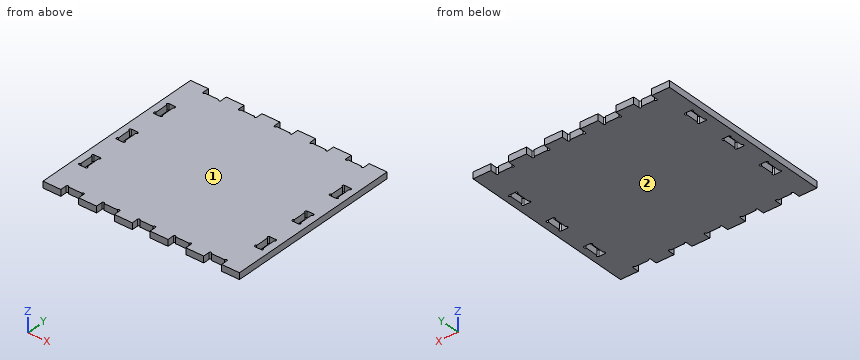
from build123d import *

# Parameters (mm, degrees)
ESTRUSIONE_ESTRUSIONE1_DEPTH = 18
TAGLIO_ESTRUSIONE1_DEPTH     = 115
TAGLIO_ESTRUSIONE2_DEPTH     = 258
TAGLIO_ESTRUSIONE3_DEPTH     = 723
TAGLIO_ESTRUSIONE4_DEPTH     = 160
TAGLIO_ESTRUSIONE5_DEPTH     = 190
TAGLIO_ESTRUSIONE6_DEPTH     = 231


with BuildPart() as part:
    # Schizzo2 → Estrusione-Estrusione1 (new body)
    with BuildSketch(Plane.XY):
        with BuildLine():
            Line((-275, -250), (-275, 250))
            Line((-275, 250), (-225, 250))
            Line((-225, 250), (-225, 232))
            ThreePointArc((-225, 232), (-221.825, 228.825), (-218.65, 232))
            Line((-218.65, 232), (-181.35, 232))
            ThreePointArc((-181.35, 232), (-178.175, 228.825), (-175, 232))
            Line((-175, 232), (-175, 250))
            Line((-175, 250), (-125, 250))
            Line((-125, 250), (-125, 232))
            ThreePointArc((-125, 232), (-121.825, 228.825), (-118.65, 232))
            Line((-118.65, 232), (-81.35, 232))
            ThreePointArc((-81.35, 232), (-78.175, 228.825), (-75, 232))
            Line((-75, 232), (-75, 250))
            Line((-75, 250), (-25, 250))
            Line((-25, 250), (-25, 232))
            ThreePointArc((-25, 232), (-21.825, 228.825), (-18.65, 232))
            Line((-18.65, 232), (18.65, 232))
            ThreePointArc((18.65, 232), (21.825, 228.825), (25, 232))
            Line((25, 232), (25, 250))
            Line((25, 250), (75, 250))
            Line((75, 250), (75, 232))
            ThreePointArc((75, 232), (78.175, 228.825), (81.35, 232))
            Line((81.35, 232), (118.65, 232))
            ThreePointArc((118.65, 232), (121.825, 228.825), (125, 232))
            Line((125, 232), (125, 250))
            Line((125, 250), (175, 250))
            Line((175, 250), (175, 232))
            ThreePointArc((175, 232), (178.175, 228.825), (181.35, 232))
            Line((181.35, 232), (218.65, 232))
            ThreePointArc((218.65, 232), (221.825, 228.825), (225, 232))
            Line((225, 232), (225, 250))
            Line((225, 250), (275, 250))
            Line((275, 250), (275, -250))
            Line((275, -250), (225, -250))
            Line((225, -250), (225, -232))
            ThreePointArc((225, -232), (221.825, -228.825), (218.65, -232))
            Line((218.65, -232), (181.35, -232))
            ThreePointArc((181.35, -232), (178.175, -228.825), (175, -232))
            Line((175, -232), (175, -250))
            Line((175, -250), (125, -250))
            Line((125, -250), (125, -232))
            ThreePointArc((125, -232), (121.825, -228.825), (118.65, -232))
            Line((118.65, -232), (81.35, -232))
            ThreePointArc((81.35, -232), (78.175, -228.825), (75, -232))
            Line((75, -232), (75, -250))
            Line((75, -250), (25, -250))
            Line((25, -250), (25, -232))
            ThreePointArc((25, -232), (21.825, -228.825), (18.65, -232))
            Line((18.65, -232), (-18.65, -232))
            ThreePointArc((-18.65, -232), (-21.825, -228.825), (-25, -232))
            Line((-25, -232), (-25, -250))
            Line((-25, -250), (-75, -250))
            Line((-75, -250), (-75, -232))
            ThreePointArc((-75, -232), (-78.175, -228.825), (-81.35, -232))
            Line((-81.35, -232), (-118.65, -232))
            ThreePointArc((-118.65, -232), (-121.825, -228.825), (-125, -232))
            Line((-125, -232), (-125, -250))
            Line((-125, -250), (-175, -250))
            Line((-175, -250), (-175, -232))
            ThreePointArc((-175, -232), (-178.175, -228.825), (-181.35, -232))
            Line((-181.35, -232), (-218.65, -232))
            ThreePointArc((-218.65, -232), (-221.825, -228.825), (-225, -232))
            Line((-225, -232), (-225, -250))
            Line((-225, -250), (-275, -250))
        make_face()
    extrude(amount=ESTRUSIONE_ESTRUSIONE1_DEPTH)

    # Schizzo2<4> → Taglio-Estrusione1 (cut)
    with BuildSketch(Plane.XY):
        with BuildLine():
            Line((237, 145.65), (237, 108.35))
            ThreePointArc((237, 108.35), (233.825, 105.175), (237, 102))
            Line((237, 102), (255, 102))
            ThreePointArc((255, 102), (258.175, 105.175), (255, 108.35))
            Line((255, 108.35), (255, 145.65))
            ThreePointArc((255, 145.65), (258.175, 148.825), (255, 152))
            Line((255, 152), (237, 152))
            ThreePointArc((237, 152), (233.825, 148.825), (237, 145.65))
        make_face()
    extrude(amount=TAGLIO_ESTRUSIONE1_DEPTH, mode=Mode.SUBTRACT)

    # Schizzo2<5> → Taglio-Estrusione2 (cut)
    with BuildSketch(Plane.XY):
        with BuildLine():
            Line((255, -18.65), (255, 18.65))
            ThreePointArc((255, 18.65), (258.175, 21.825), (255, 25))
            Line((255, 25), (237, 25))
            ThreePointArc((237, 25), (233.825, 21.825), (237, 18.65))
            Line((237, 18.65), (237, -18.65))
            ThreePointArc((237, -18.65), (233.825, -21.825), (237, -25))
            Line((237, -25), (255, -25))
            ThreePointArc((255, -25), (258.175, -21.825), (255, -18.65))
        make_face()
    extrude(amount=TAGLIO_ESTRUSIONE2_DEPTH, mode=Mode.SUBTRACT)

    # Schizzo2<7> → Taglio-Estrusione3 (cut)
    with BuildSketch(Plane.XY):
        with BuildLine():
            Line((255, -152), (237, -152))
            ThreePointArc((237, -152), (233.825, -148.825), (237, -145.65))
            Line((237, -145.65), (237, -108.35))
            ThreePointArc((237, -108.35), (233.825, -105.175), (237, -102))
            Line((237, -102), (255, -102))
            ThreePointArc((255, -102), (258.175, -105.175), (255, -108.35))
            Line((255, -108.35), (255, -145.65))
            ThreePointArc((255, -145.65), (258.175, -148.825), (255, -152))
        make_face()
    extrude(amount=TAGLIO_ESTRUSIONE3_DEPTH, mode=Mode.SUBTRACT)

    # Schizzo2<8> → Taglio-Estrusione4 (cut)
    with BuildSketch(Plane.XY):
        with BuildLine():
            Line((-255, 152), (-237, 152))
            ThreePointArc((-237, 152), (-233.825, 148.825), (-237, 145.65))
            Line((-237, 145.65), (-237, 108.35))
            ThreePointArc((-237, 108.35), (-233.825, 105.175), (-237, 102))
            Line((-237, 102), (-255, 102))
            ThreePointArc((-255, 102), (-258.175, 105.175), (-255, 108.35))
            Line((-255, 108.35), (-255, 145.65))
            ThreePointArc((-255, 145.65), (-258.175, 148.825), (-255, 152))
        make_face()
    extrude(amount=TAGLIO_ESTRUSIONE4_DEPTH, mode=Mode.SUBTRACT)

    # Schizzo2<9> → Taglio-Estrusione5 (cut)
    with BuildSketch(Plane.XY):
        with BuildLine():
            Line((-255, 25), (-237, 25))
            ThreePointArc((-237, 25), (-233.825, 21.825), (-237, 18.65))
            Line((-237, 18.65), (-237, -18.65))
            ThreePointArc((-237, -18.65), (-233.825, -21.825), (-237, -25))
            Line((-237, -25), (-255, -25))
            ThreePointArc((-255, -25), (-258.175, -21.825), (-255, -18.65))
            Line((-255, -18.65), (-255, 18.65))
            ThreePointArc((-255, 18.65), (-258.175, 21.825), (-255, 25))
        make_face()
    extrude(amount=TAGLIO_ESTRUSIONE5_DEPTH, mode=Mode.SUBTRACT)

    # Schizzo2<10> → Taglio-Estrusione6 (cut)
    with BuildSketch(Plane.XY):
        with BuildLine():
            Line((-237, -145.65), (-237, -108.35))
            ThreePointArc((-237, -108.35), (-233.825, -105.175), (-237, -102))
            Line((-237, -102), (-255, -102))
            ThreePointArc((-255, -102), (-258.175, -105.175), (-255, -108.35))
            Line((-255, -108.35), (-255, -145.65))
            ThreePointArc((-255, -145.65), (-258.175, -148.825), (-255, -152))
            Line((-255, -152), (-237, -152))
            ThreePointArc((-237, -152), (-233.825, -148.825), (-237, -145.65))
        make_face()
    extrude(amount=TAGLIO_ESTRUSIONE6_DEPTH, mode=Mode.SUBTRACT)


solid = part.part
Work out the finished part from the listing and answer in its coordinate system (mm). Face numbers are marked on the shaded views. Give positions to 0.01 mm unless a question says otherwise; leave off trailing zeros. Loops run counter-clockwise (first coordinate to the right, second up) from the corner with the lowest first, then second, coordinate; pieces in that order, holes last. Notation, with made-up numbers: (29, -21) - (86, -21) arc R21 ccw to (86, 17) - close; hole circle Ø8 at (-23, -4). An arc over 180 degrees is marked (long way). Answer in a Markdown table with one row per item.
(1) Consider L1, parallel to X at y = -133, z = 4.25; L2, parallel to Y at x = 240.5, z = 14.75; L3, parallel to X at y = -105.5, z = 14.75. Determine where each line is inside the solid, lowest interval first. Write a range as [from, to].
Results list:
| item | result |
|---|---|
| L1 | x = [-275, -255], [-237, 237], [255, 275] |
| L2 | y = [-250, -152], [-102, -25], [25, 102], [152, 250] |
| L3 | x = [-275, -258.16], [-233.84, 233.84], [258.16, 275] |
(2) For a pull along Z with two mould halves and no side action, classify the marked faces 1 and 2 as pulls with the +Z half, pulls with the -Z half, needs draft (parallel to the pull), parting line crosses it, or undercut.
Results list:
| item | result |
|---|---|
| face 1 | pulls with the +Z half |
| face 2 | pulls with the -Z half |
(3) A flat-ended cylindrical pin translates along its axis: pin 1 Ø6 at (x, z) = (-1, 15.5) entering from +Y. Find the tip coordinate at first contact, or state that the pin passes through.
Results list:
| item | result |
|---|---|
| pin 1 | stops at y = 232 |
(4) Section A-A (z = 9.75) is taken. State how many separate pieces and enclosed holes the cut face has, and give its area (3 significant figures).
Results list:
| item | result |
|---|---|
| separate pieces | 1 |
| enclosed holes | 6 |
| area | 260,000 mm² |
(5) Section B-B (x = 99.5) is taken. Give the vertices of the cut face in (y, z), and give its area (3 significant figures).
Results list:
| item | result |
|---|---|
| outline | (-232, 0) - (232, 0) - (232, 18) - (-232, 18) - close |
| area | 8,350 mm² |
